```python
from build123d import *

# Parameters (mm, degrees)
SKETCH1_W           = 60
SKETCH1_H           = 75
BOSS_EXTRUDE1_DEPTH = 20
SKETCH2_W           = 18.666666667
SKETCH2_H           = 73
CUT_EXTRUDE1_DEPTH  = 19
SKETCH3_W           = 18.666666666
SKETCH3_H           = 73
CUT_EXTRUDE2_DEPTH  = 19
SKETCH4_W           = 18.666666667
SKETCH4_H           = 73
CUT_EXTRUDE3_DEPTH  = 19


with BuildPart() as part:
    # Sketch1 → Boss-Extrude1 (new body)
    with BuildSketch(Plane.XY):
        Rectangle(SKETCH1_W, SKETCH1_H)
    extrude(amount=-BOSS_EXTRUDE1_DEPTH)

    # Sketch2 → Cut-Extrude1 (cut)
    with BuildSketch(Plane.XY):
        with Locations((-19.666666667, 0)):
            Rectangle(SKETCH2_W, SKETCH2_H)
    extrude(amount=-CUT_EXTRUDE1_DEPTH, mode=Mode.SUBTRACT)

    # Sketch3 → Cut-Extrude2 (cut)
    with BuildSketch(Plane.XY):
        Rectangle(SKETCH3_W, SKETCH3_H)
    extrude(amount=-CUT_EXTRUDE2_DEPTH, mode=Mode.SUBTRACT)

    # Sketch4 → Cut-Extrude3 (cut)
    with BuildSketch(Plane.XY):
        with Locations((19.666666667, 0)):
            Rectangle(SKETCH4_W, SKETCH4_H)
    extrude(amount=-CUT_EXTRUDE3_DEPTH, mode=Mode.SUBTRACT)


solid = part.part
```
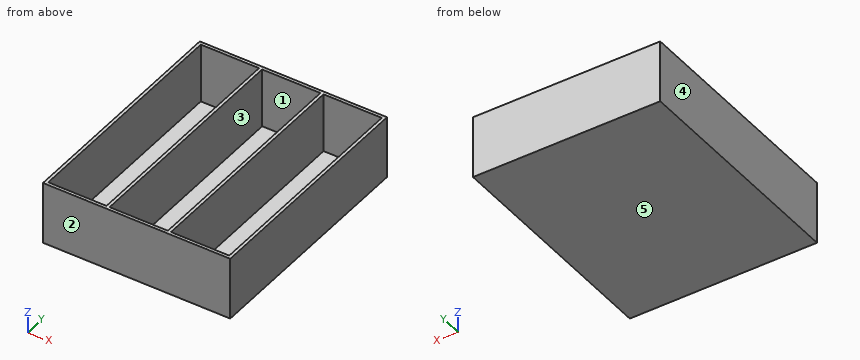
The model under review builds one solid part; all positions refer to its coordinate system, in mm. Face numbers are marked on the shaded views. A direction names the side the tool comes from. Give positions to 0.01 mm unless a question says otherwise; leave off trailing zeros. Write each loop counter-clockwise with the first axis right and the second up, starting at its lowest first coordinate (ties: lowest second). Pieces come first, ordered by that corner, then holes. Notation, with made-up numbers: (-3, 20) - (39, 20) arc R20 ccw to (39, 28) - close; hole circle Ø7 at (72, 23). An arc over 180 degrees is marked (long way). Answer in a Markdown table with one row per item. Add a question column.
1. Insertion check: P1, Ø5.5, axis at x = -0.5, y = 7.5, coming from the +Z side. The pin has a flat end and moves straight along its axis. Give the tip position at first contact, or say it passes through.
2. Wall thickness on line 1 along X through (y, z) = (-18.5, -5.5); line 2 along Y through (x, z) = (-18, -14.25); line 3 along Z through (x, y) = (13.5, 28.5): over which ranges is each line inside the solid? List them lowest first. Write a range as [from, to].
3. We need section B-B on y = 28. Write out the cut boundary in (x, z), then the cut area to 3 significant figures.
4. Draft analysis for pull direction X (two halves, no side actions). For the marked faces 3, 4 and 5, state which applies: +X half, -X half, draft (parallel to the pull), parting line (faces both ways), or undercut.
5. We need section C-C on x = 4. Write out the cut boundary in (y, z), then the cut area to 3 significant figures.
6. Tool access review of the marked faces 1 and 2: name each direction out of +Z, -Z, +X, -X, +Y, -Y from which nothing blocks a thin tool from reaching the whole face with its end or side.
7. We need section A-A on z = -7.75. Write out the cut boundary in (x, y), then the cut area to 3 significant figures.
Ans:
| question | item | result |
|---|---|---|
| 1 | P1 | stops at z = -19 |
| 2 | line 1 | x = [-30, -29], [-10.33, -9.33], [9.33, 10.33], [29, 30] |
| 2 | line 2 | y = [-37.5, -36.5], [36.5, 37.5] |
| 2 | line 3 | z = [-20, -19] |
| 3 | outline | (-30, -20) - (30, -20) - (30, 0) - (29, 0) - (29, -19) - (10.33, -19) - (10.33, 0) - (9.33, 0) - (9.33, -19) - (-9.33, -19) - (-9.33, 0) - (-10.33, 0) - (-10.33, -19) - (-29, -19) - (-29, 0) - (-30, 0) - close |
| 3 | area | 136 mm^2 |
| 4 | face 3 | undercut |
| 4 | face 4 | -X half |
| 4 | face 5 | draft |
| 5 | outline | (-37.5, -20) - (37.5, -20) - (37.5, 0) - (36.5, 0) - (36.5, -19) - (-36.5, -19) - (-36.5, 0) - (-37.5, 0) - close |
| 5 | area | 113 mm^2 |
| 6 | face 1 | +Z |
| 6 | face 2 | +Z, -Z, +X, -X, -Y |
| 7 | outline | (-30, -37.5) - (30, -37.5) - (30, 37.5) - (-30, 37.5) - close; hole (-29, -36.5) - (-10.33, -36.5) - (-10.33, 36.5) - (-29, 36.5) - close; hole (-9.33, -36.5) - (9.33, -36.5) - (9.33, 36.5) - (-9.33, 36.5) - close; hole (10.33, -36.5) - (29, -36.5) - (29, 36.5) - (10.33, 36.5) - close |
| 7 | area | 412 mm^2 |
